```python
from build123d import *

# Parameters (mm, degrees)
SKETCH1_R           = 11
BOSS_EXTRUDE1_DEPTH = 36
EXTRUDE_THIN1_START = 0.5
SKETCH1_4_R         = 6.5
SKETCH1_4_R_2       = 6
EXTRUDE_THIN1_DEPTH = 29.5
BOSS_EXTRUDE2_START = 0.8
SKETCH1_5_R         = 10
SKETCH1_5_R_2       = 6
BOSS_EXTRUDE2_DEPTH = 29
BOSS_EXTRUDE3_START = 0.3
SKETCH1_6_R         = 11
SKETCH1_6_R_2       = 10
BOSS_EXTRUDE3_DEPTH = 31
BOSS_EXTRUDE4_START = 1
BOSS_EXTRUDE4_DEPTH = 1
FILLET1_R           = 0.5
SKETCH4_R           = 2.15
CUT_EXTRUDE3_DEPTH  = 51.209560914
CHAMFER1_SIZE       = 1


with BuildPart() as part:
    # Sketch1 → Boss-Extrude1 (new body)
    with BuildSketch(Plane(origin=(0, 0, 0), x_dir=(0, 0, -1), z_dir=(1, 0, 0))):
        Polygon((-21, -7), (-19.5, -5.5), (-19.5, 9), (-11, 9), (-5, 13), (5, 13), (11, 9), (19.5, 9), (19.5, -5.5), (21, -7), (21, -15), (11, -15), (9.5, -13.5), (-9.5, -13.5), (-11, -15), (-21, -15), align=None)
        Circle(SKETCH1_R, mode=Mode.SUBTRACT)
    extrude(amount=BOSS_EXTRUDE1_DEPTH)



with BuildPart() as body_2:
    # Sketch1_4 → Extrude-Thin1 (new body)
    with BuildSketch(Plane(origin=(0, 0, 0), x_dir=(0, 0, -1), z_dir=(1, 0, 0)).offset(EXTRUDE_THIN1_START)):
        Circle(SKETCH1_4_R)
        Circle(SKETCH1_4_R_2, mode=Mode.SUBTRACT)
    extrude(amount=EXTRUDE_THIN1_DEPTH)

    # Sketch1_5 → Boss-Extrude2 (add)
    with BuildSketch(Plane(origin=(0, 0, 0), x_dir=(0, 0, -1), z_dir=(1, 0, 0)).offset(BOSS_EXTRUDE2_START)):
        with Locations(Location((0, 0, 0), (0, 0, 180))):
            Circle(SKETCH1_5_R)
        Circle(SKETCH1_5_R_2, mode=Mode.SUBTRACT)
    extrude(amount=BOSS_EXTRUDE2_DEPTH)


with BuildPart() as part_1:
    add(part.part)

    add(body_2.part)  # Boss-Extrude3 merges body 2
    # Sketch1_6 → Boss-Extrude3 (add)
    with BuildSketch(Plane(origin=(0, 0, 0), x_dir=(0, 0, -1), z_dir=(1, 0, 0)).offset(BOSS_EXTRUDE3_START)):
        Circle(SKETCH1_6_R)
        Circle(SKETCH1_6_R_2, mode=Mode.SUBTRACT)
    extrude(amount=BOSS_EXTRUDE3_DEPTH)

    # Sketch3 → Boss-Extrude4 (add)
    with BuildSketch(Plane(origin=(31.3, 0, 0), x_dir=(0, 0, -1), z_dir=(1, 0, 0)).offset(BOSS_EXTRUDE4_START)):
        with BuildLine():
            Line((-1.011429614, -9.94871902), (-1.112572576, -10.943590922))
            ThreePointArc((-1.112572576, -10.943590922), (0, 11), (1.112572576, -10.943590922))
            Line((1.112572576, -10.943590922), (1.011429614, -9.94871902))
            ThreePointArc((1.011429614, -9.94871902), (1.535872296, -8.912190675), (2.686623353, -9.070945649))
            ThreePointArc((2.686623353, -9.070945649), (4.301522401, -8.715825098), (3.378506843, -7.343946161))
            ThreePointArc((3.378506843, -7.343946161), (0, 8.083801933), (-3.378506843, -7.343946161))
            ThreePointArc((-3.378506843, -7.343946161), (-4.301522401, -8.715825098), (-2.686623353, -9.070945649))
            ThreePointArc((-2.686623353, -9.070945649), (-1.535872296, -8.912190675), (-1.011429614, -9.94871902))
        make_face()
    extrude(amount=BOSS_EXTRUDE4_DEPTH)

    # Fillet1
    fillet1_edges = [part_1.edges().sort_by_distance(p)[0] for p in [
        (36, -6.25, 20.25),
        (36, -11, 21),
        (0, 1.75, 19.5),
        (0, 9, 15.25),
        (0, 11, 8),
        (0, 13, 0),
        (0, 11, -8),
        (0, 9, -15.25),
        (0, 1.75, -19.5),
        (0, -6.25, -20.25),
        (0, -11, -21),
        (0, -11, 21),
        (0, -6.25, 20.25),
        (18, -5.5, 19.5),
        (18, 9, 19.5),
        (18, 9, 11),
        (18, 13, 5),
        (18, 13, -5),
        (18, 9, -11),
        (18, 9, -19.5),
        (18, -5.5, -19.5),
        (18, -7, -21),
        (18, -7, 21),
        (36, -11, -21),
        (36, -6.25, -20.25),
        (36, 1.75, -19.5),
        (36, 9, -15.25),
        (36, 11, -8),
        (36, 13, 0),
        (36, 11, 8),
        (36, 9, 15.25),
        (36, 1.75, 19.5),
    ]]
    fillet(fillet1_edges, radius=FILLET1_R)

    # Sketch4 → Cut-Extrude3 (cut, through all)
    with BuildSketch(Plane.XZ.offset(15)):
        with Locations(Location((5, 15.25, 0), (0, 0, 270))):
            Circle(SKETCH4_R)
        with Locations(Location((31, 15.25, 0), (0, 0, 270))):
            Circle(SKETCH4_R)
        with Locations(Location((31, -15.25, 0), (0, 0, 270))):
            Circle(SKETCH4_R)
        with Locations(Location((5, -15.25, 0), (0, 0, 270))):
            Circle(SKETCH4_R)
    extrude(amount=-CUT_EXTRUDE3_DEPTH, mode=Mode.SUBTRACT)

    # Chamfer1
    chamfer1_edges = [part_1.edges().sort_by_distance(p)[0] for p in [
        (5, 9, -13.1),
        (5, -15, -13.1),
        (31, 9, -13.1),
        (31, -15, -13.1),
        (31, 9, 17.4),
        (31, -15, 17.4),
        (5, 9, 17.4),
        (5, -15, 17.4),
    ]]
    chamfer(chamfer1_edges, length=CHAMFER1_SIZE)


solid = part_1.part
```
Source: CAD feature listing. Evaluate the final solid. Frame: model axes, mm. A direction names the side the tool comes from. Coordinates: 2 decimals unless noted, no trailing zeros. Write each loop counter-clockwise with the first axis right and the second up, starting at its lowest first coordinate (ties: lowest second). Pieces come first, ordered by that corner, then holes. Notation, with made-up numbers: (46.25, 6) - (67.25, 6) arc R18 cw to (67.25, 33) - close; hole circle Ø8 at (81.5, 23.25). An arc over 180 degrees is marked (long way). Answer as a JSON object with one key per item and string values.
Q1. Material intervals for line 1 (X direction, y = 1.75, z = -15.25); line 2 (Z direction, x = 32, y = -5); line 3 (X direction, y = 8.75, z = -17), sorted ascending. Write a range as [from, to].
Ans:
{"line 1": "x = [0, 2.85], [7.15, 28.85], [33.15, 36]", "line 2": "z = [-19.5, -17.15], [-13.35, -9.8], [9.8, 13.35], [17.15, 19.5]", "line 3": "x = [0.07, 2.69], [7.31, 28.69], [33.31, 35.93]"}
Q2. Section query C-C, the plane x = 5. State how many separate pieces and enclosed holes the cut face has, plus the area to 3 significant figures.
Ans:
{"separate pieces": "3", "enclosed holes": "1", "area": "672 mm2"}
Q3. Draft query along Z for faces 5 (the flat face through (18, -6, 20)), 6 (the cylindrical face through (33.617, -4.213, -10.161)), 7 (the flat face through (0, -10, -5)). Return one class per face: released by +Z, released by -Z, zero draft, split by the parting line, or undercut.
Ans:
{"face 5": "released by +Z", "face 6": "undercut", "face 7": "zero draft"}
Q4. First-contact query: pin 1 Ø6.5 at (y, z) = (2, 1) entering from -X; pin 2 Ø15 at (x, y) = (17.5, 3) entering from +Z; pin 3 Ø4 at (x, z) = (25.5, 14) entering from +Y; pin 4 Ø4 at (x, y) = (23, 2.5) entering from -Z. Flat tips, straight axial feed; report the tip coordinate or a pass-through.
Ans:
{"pin 1": "passes through", "pin 2": "stops at z = 19.5", "pin 3": "stops at y = 9", "pin 4": "stops at z = -19.5"}
Q5. Section query A-A, the plane z = 15.25. Output: boundary loops of the cut face in (x, y), plus the area to 3 significant figures.
Ans:
{"outline": "(0, -15) - (1.85, -15) - (2.85, -14) - (2.85, 8) - (1.85, 9) - (0.5, 9) arc R0.5 ccw to (0, 8.5) - close; (7.15, -14) - (8.15, -15) - (27.85, -15) - (28.85, -14) - (28.85, 8) - (27.85, 9) - (8.15, 9) - (7.15, 8) - close; (33.15, -14) - (34.15, -15) - (36, -15) - (36, 8.5) arc R0.5 ccw to (35.5, 9) - (34.15, 9) - (33.15, 8) - close", "area": "653 mm2"}
Q6. Section query B-B, the plane x = 15. Output: boundary loops of the cut face in (y, z), plus the area to 3 significant figures.
Ans:
{"outline": "(-15, -21) - (-7.21, -21) arc R0.5 ccw to (-6.85, -20.85) - (-5.65, -19.65) arc R0.5 cw to (-5.29, -19.5) - (8.5, -19.5) arc R0.5 ccw to (9, -19) - (9, -11.15) arc R0.5 cw to (9.08, -10.87) - (12.92, -5.13) arc R0.5 ccw to (13, -4.85) - (13, 4.85) arc R0.5 ccw to (12.92, 5.13) - (9.08, 10.87) arc R0.5 cw to (9, 11.15) - (9, 19) arc R0.5 ccw to (8.5, 19.5) - (-5.29, 19.5) arc R0.5 cw to (-5.65, 19.65) - (-6.85, 20.85) arc R0.5 ccw to (-7.21, 21) - (-15, 21) - (-15, 11) - (-13.5, 9.5) - (-13.5, -9.5) - (-15, -11) - close; hole circle Ø12 at (0, 0)", "area": "882 mm2"}
Q7. Set-up query: faces 1 (the cylindrical face through (32.81, -3.15, -16.41)), 2 (the flat face through (31.3, -10, -2)), 3 (the flat face through (30, -6, -2)), 4 (the flat face through (18, -14, 10)). Return all of +Z, -Z, +X, -X, +Y, -Y with unobstructed straight access to the full face (end or side cutting, diameter ignored); none if empty.
Ans:
{"face 1": "+Y, -Y", "face 2": "none", "face 3": "+X", "face 4": "+X, -X, -Y"}
